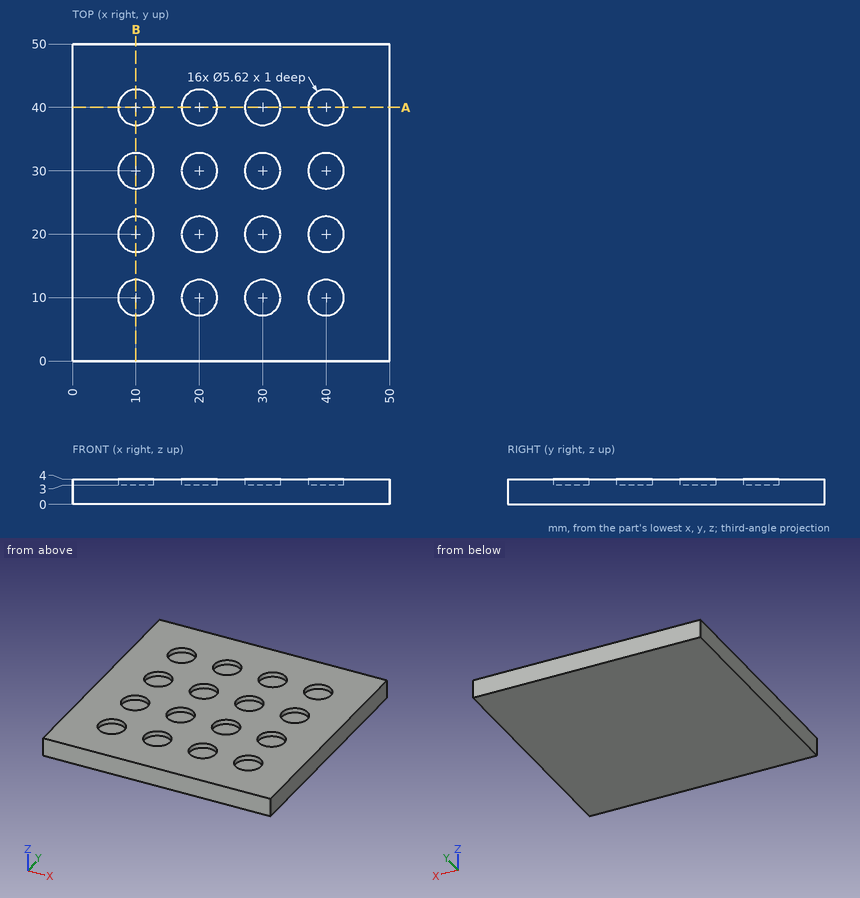
Could you check a few things on this drawing? It's one solid part, dimensions in mm from its lowest x, y, z. Coordinates: 2 decimals unless noted, no trailing zeros. Write each loop counter-clockwise with the first axis right and the second up, starting at its lowest first coordinate (ties: lowest second). Pieces come first, ordered by that corner, then holes.
Q1. Imagine slicing it at A-A, the plane y = 40. List the corners of the cut face in (x, z) for me.
Results found:
outline: (0, 0) - (50, 0) - (50, 4) - (42.81, 4) - (42.81, 3) - (37.19, 3) - (37.19, 4) - (32.81, 4) - (32.81, 3) - (27.19, 3) - (27.19, 4) - (22.81, 4) - (22.81, 3) - (17.19, 3) - (17.19, 4) - (12.81, 4) - (12.81, 3) - (7.19, 3) - (7.19, 4) - (0, 4) - close
Q2. Please list where these lines run through material, in increasing order: L1, parallel to Y at x = 40, z = 3.35; L2, parallel to Z at x = 28.5, y = 8.
Results found:
L1: y = 0 to 7.19, 12.81 to 17.19, 22.81 to 27.19, 32.81 to 37.19, 42.81 to 50
L2: z = 0 to 3
Q3. For P1, Ø4.5, axis at x = 10, y = 40.5, coming from the +Z side, with a flat end and sliding along its axis, tell me the tip position at first contact or that it passes through.
Results found:
P1: stops at z = 3
